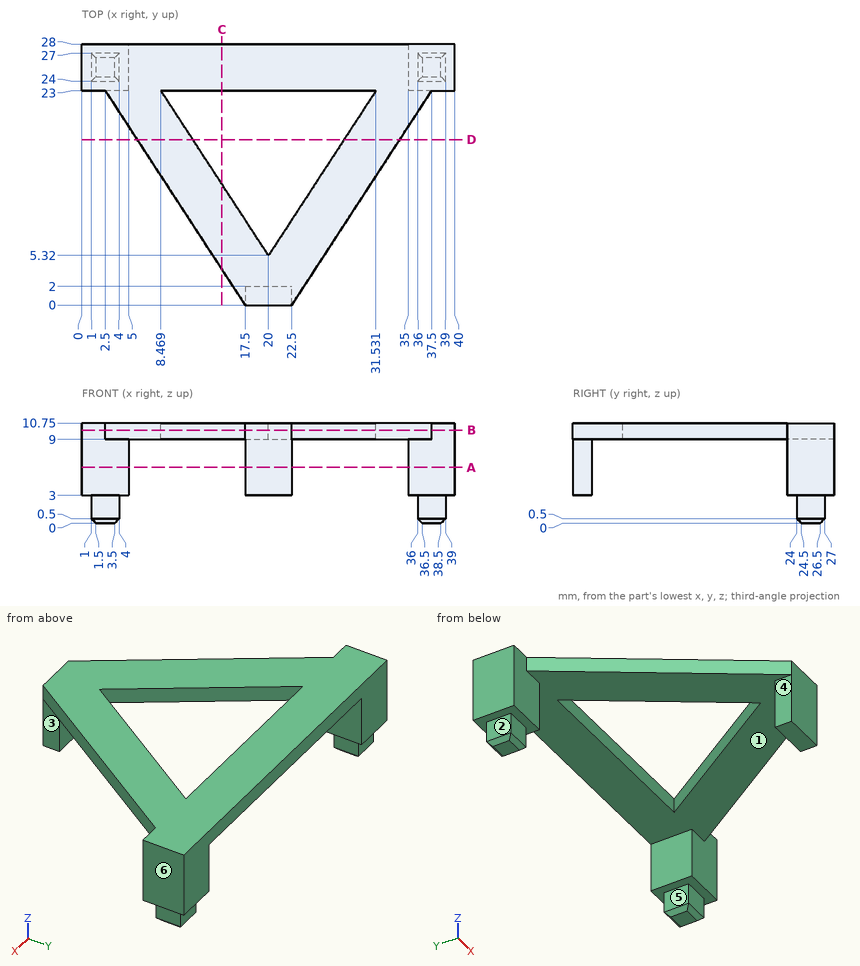
Geometry check sheet. Reference: drawing and pictorial views, mm from the part's lowest x, y, z. A direction names the side the tool comes from. Give positions to 0.01 mm unless a question says otherwise; leave off trailing zeros. Write each loop counter-clockwise with the first axis right and the second up, starting at its lowest first coordinate (ties: lowest second). Pieces come first, ordered by that corner, then holes.
Item 1: Gauge pin test, flat ends, axial feed: pin 1 (5 mm diameter, centred on x = 17.5, y = 23.5, fed in from -Z); pin 2 (2 mm diameter, centred on y = 1.5, z = 6.5, fed in from +X); pin 3 (5 mm diameter, centred on x = 8, z = 2.5, fed in from -Y); pin 4 (1 mm diameter, centred on y = 16.5, z = 9.5, fed in from -X). Record the tip position at first contact, or that the pin passes through.
Item 2: Cross-section at B-B (z = 10). Enter the section's corners in (x, y), and give its area (3 significant figures).
Item 3: Draft check along X on the marked faces 1, 2 and 3. Enter one of: released by +X, released by -X, zero draft, split by the parting line, or undercut.
Item 4: Cross-section at C-C (x = 15). Enter the section's corners in (y, z).
Item 5: Cross-section at A-A (z = 6). Enter the section's corners in (x, y), and give its area (3 significant figures).
Item 6: Access from +Z, -Z, +X, -X, +Y, -Y to the whole of each face (thin tool, end or side, straight path). Record for the marked faces 4, 5 and 6.
Item 7: Cross-section at D-D (y = 17.75). Enter the section's corners in (x, z), and give its area (3 significant figures).
Item 8: Scan lines: L1, parallel to X at y = 24.75, z = 5.75; L2, parallel to Z at x = 25.5, y = 25.75; L3, parallel to Y at x = 22, z = 3.25. Record each from-to range of solid material in increasing order.
Report:
1. pin 1: stops at z = 9
1. pin 2: stops at x = 22.5
1. pin 3: passes through
1. pin 4: stops at x = 6.41
2. outline: (0, 23) - (2.5, 23) - (17.5, 0) - (22.5, 0) - (37.5, 23) - (40, 23) - (40, 28) - (0, 28) - close; hole (8.47, 23) - (20, 5.32) - (31.53, 23) - close
2. area: 456 mm2
3. face 1: undercut
3. face 2: released by -X
3. face 3: released by +X
4. outline: (3.83, 9) - (12.99, 9) - (12.99, 10.75) - (3.83, 10.75) - close; (23, 9) - (28, 9) - (28, 10.75) - (23, 10.75) - close
5. outline: (0, 23) - (5, 23) - (5, 28) - (0, 28) - close; (17.5, 0) - (22.5, 0) - (22.5, 2) - (17.5, 2) - close; (35, 23) - (40, 23) - (40, 28) - (35, 28) - close
5. area: 60.0 mm2
6. face 4: -Z, -X, +Y, -Y
6. face 5: -Z, +Y, -Y
6. face 6: +Z, -Z, +X, +Y, -Y
7. outline: (5.92, 9) - (11.89, 9) - (11.89, 10.75) - (5.92, 10.75) - close; (28.11, 9) - (34.08, 9) - (34.08, 10.75) - (28.11, 10.75) - close
7. area: 20.9 mm2
8. L1: x = 0 to 5, 35 to 40
8. L2: z = 9 to 10.75
8. L3: y = 0 to 2
